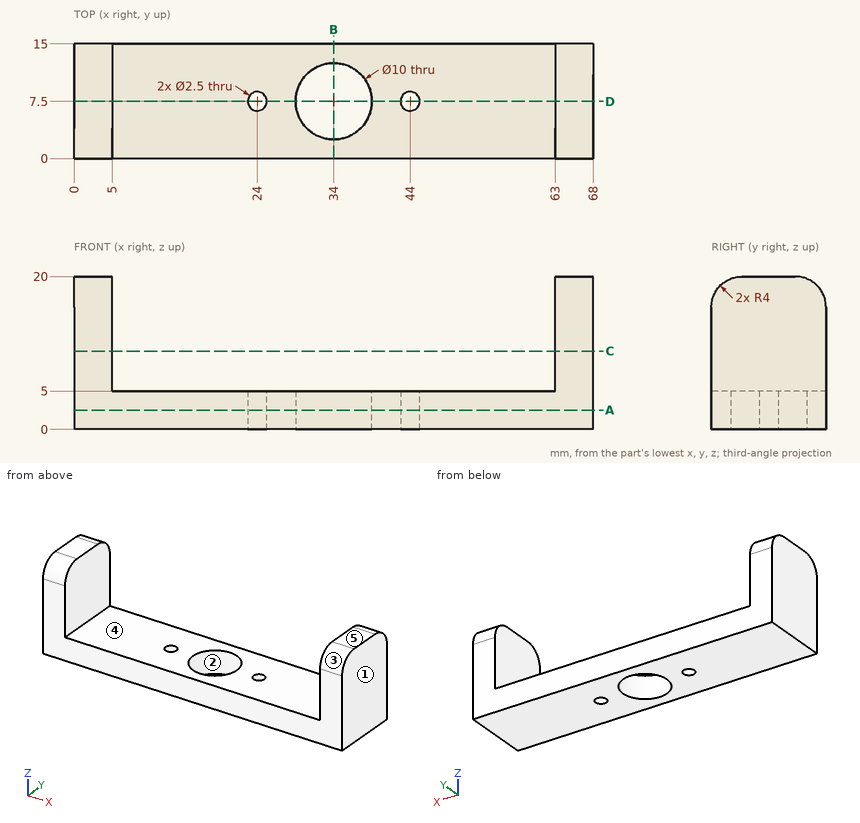
Answer from the drawing. Dimensions are ordinates in mm from the lowest x, y and z of the part. A direction names the side the tool comes from. Give positions to 0.01 mm unless a question says otherwise; leave off trailing zeros. Order: outer loops, then holes, each group sorted by start corner. A loop starts at its lowest first (then second) coordinate and runs counter-clockwise, first axis right, second up. Notation, with made-up numbers: (59.5, 35) - (91.5, 35) arc R29 cw to (91.5, 74) - close; hole circle Ø5 at (72.5, -23). An arc over 180 degrees is marked (long way). Use one line per item in the form item = value.
1) Find section C-C on z = 10.25. Determine the outline of the cut face in (x, y).
Verdict:
outline = (0, 0) - (5, 0) - (5, 15) - (0, 15) - close; (63, 0) - (68, 0) - (68, 15) - (63, 15) - close
2) The mould has two halves that part along Y. Classify the marked faces 1, 2 and 3: released by +Y, released by -Y, zero draft, split by the parting line, or undercut.
Verdict:
face_1 = zero draft
face_2 = undercut
face_3 = released by -Y
3) Each of these flat-tipped pins is pushed along its axis until it touches: pin 1 (2 mm diameter, centred on x = 29.5, z = 2, fed in from -Y); pin 2 (7.5 mm diameter, centred on x = 28.5, y = 9, fed in from +Z). Where does it stop, or does it pass through?
Verdict:
pin_1 = 0
pin_2 = 5
4) Find section B-B on x = 34. Determine the outline of the cut face in (y, z).
Verdict:
outline = (0, 0) - (2.5, 0) - (2.5, 5) - (0, 5) - close; (12.5, 0) - (15, 0) - (15, 5) - (12.5, 5) - close
5) Find section A-A on z = 2.5. Determine the outline of the cut face in (x, y), and give its area (3 significant figures).
Verdict:
outline = (0, 0) - (68, 0) - (68, 15) - (0, 15) - close; hole circle Ø2.5 at (24, 7.5); hole circle Ø10 at (34, 7.5); hole circle Ø2.5 at (44, 7.5)
area = 932 mm^2
6) Consider probe 1 along X at (y, z) = (4, 11.25); probe 2 along Y at (x, z) = (44, 3.25); probe 3 along Z at (x, y) = (58, 13.5). Determine where each line is inside the solid, lowest interval first. Write a range as [from, to].
Verdict:
probe_1 = [0, 5], [63, 68]
probe_2 = [0, 6.25], [8.75, 15]
probe_3 = [0, 5]
7) Find section D-D on y = 7.5. Determine the outline of the cut face in (x, z), and give its area (3 significant figures).
Verdict:
outline = (0, 0) - (22.75, 0) - (22.75, 5) - (5, 5) - (5, 20) - (0, 20) - close; (25.25, 0) - (29, 0) - (29, 5) - (25.25, 5) - close; (39, 0) - (42.75, 0) - (42.75, 5) - (39, 5) - close; (45.25, 0) - (68, 0) - (68, 20) - (63, 20) - (63, 5) - (45.25, 5) - close
area = 415 mm^2
8) For the marked faces 4 and 5, determine the directions among +Z, -Z, +X, -X, +Y, -Y from which every point of the face is accessible in a straight line to the end or side of a thin tool.
Verdict:
face_4 = +Z, +Y, -Y
face_5 = +Z, +X, -X, +Y, -Y
